Could you check a few things on this drawing? It's one solid part, dimensions in mm from its lowest x, y, z. Round coordinates to 2 decimals unless told otherwise and drop trailing zeros. Write each loop counter-clockwise with the first axis right and the second up, starting at its lowest first coordinate (ties: lowest second). Pieces come first, ordered by that corner, then holes. Notation, with made-up numbers: (20, -19.75) - (63, -19.75) arc R27 cw to (63, 8.25) - close; hole circle Ø9 at (-5.75, 24.5). An arc over 180 degrees is marked (long way). Use one line per item in the form item = value. Start each with the question number.
1. I want a section at A-A, the plane x = 10.5. List the corners of the cut face in (y, z) for me (1 decimal).
2. Will these pins go through, and if not, where does the flat tip stop? pin 1 (1.5 mm diameter, centred on y = 0.5, z = 26, fed in from +X); pin 2 (1 mm diameter, centred on x = 11, y = 1, fed in from +Z) (1 decimal); pin 3 (1 mm diameter, centred on y = 0.5, z = 59, fed in from -X).
3. If I drill on line 1 along Z through (x, y) = (20.5, 2.45) (1 decimal); line 2 along Z through (x, y) = (40, 1.25) (1 decimal); line 3 along Z through (x, y) = (31, 2) (1 decimal), over which ranges is the centre line in solid material (lowest first)?
4. I want a section at B-B, the plane x = 22. List the corners of the cut face in (y, z) for me.
5. I want a section at D-D, the plane x = 43.5. List the corners of the cut face in (y, z) for me (1 decimal).
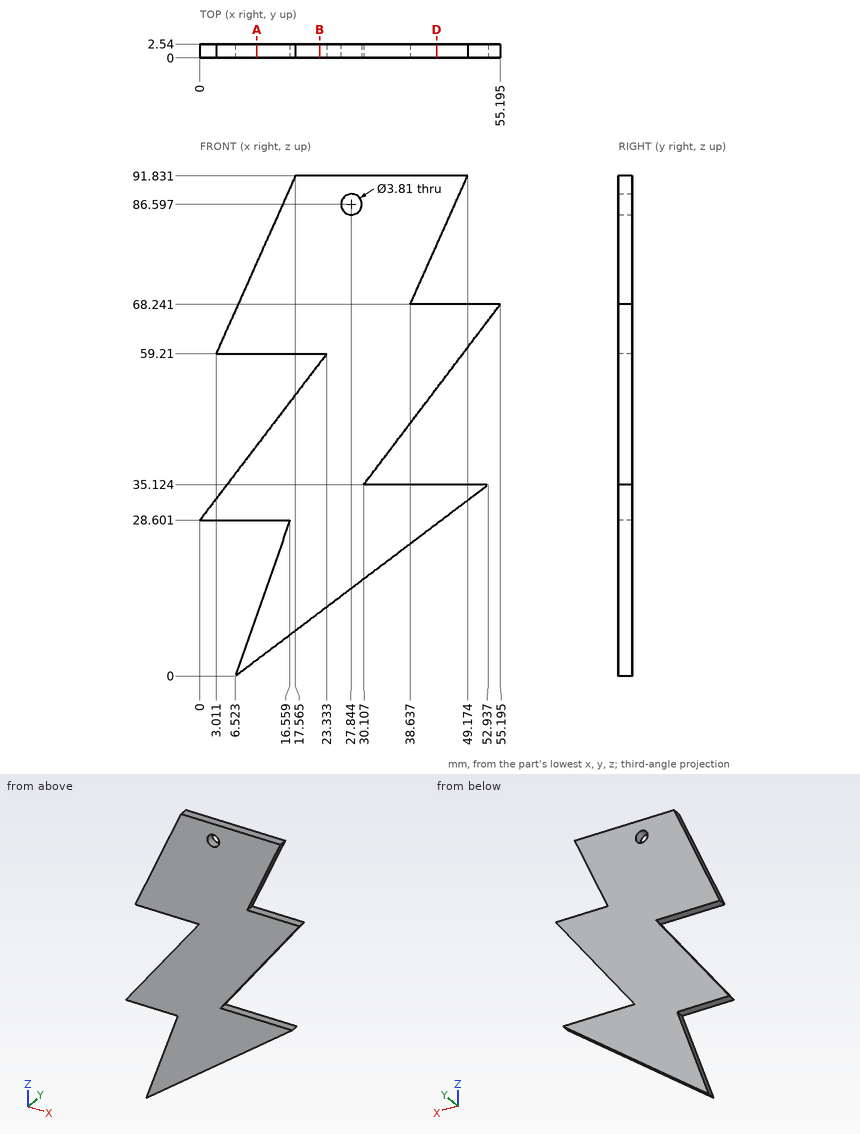
Model answer:
q1.outline = (0, 3) - (2.5, 3) - (2.5, 11.3) - (0, 11.3) - close; (0, 28.6) - (2.5, 28.6) - (2.5, 42.4) - (0, 42.4) - close; (0, 59.2) - (2.5, 59.2) - (2.5, 76) - (0, 76) - close
q2.pin_1 = 41.87
q2.pin_2 = 78.2
q2.pin_3 = 3.01
q3.line_1 = 10.6 to 55.5, 59.2 to 91.8
q3.line_2 = 25.3 to 35.1, 48.2 to 68.2, 71.3 to 91.8
q3.line_3 = 18.5 to 35.1, 36.3 to 91.8
q4.outline = (0, 11.71) - (2.54, 11.71) - (2.54, 57.46) - (0, 57.46) - close; (0, 59.21) - (2.54, 59.21) - (2.54, 91.83) - (0, 91.83) - close
q5.outline = (0, 28) - (2.5, 28) - (2.5, 35.1) - (0, 35.1) - close; (0, 52.8) - (2.5, 52.8) - (2.5, 68.2) - (0, 68.2) - close; (0, 79.1) - (2.5, 79.1) - (2.5, 91.8) - (0, 91.8) - close
